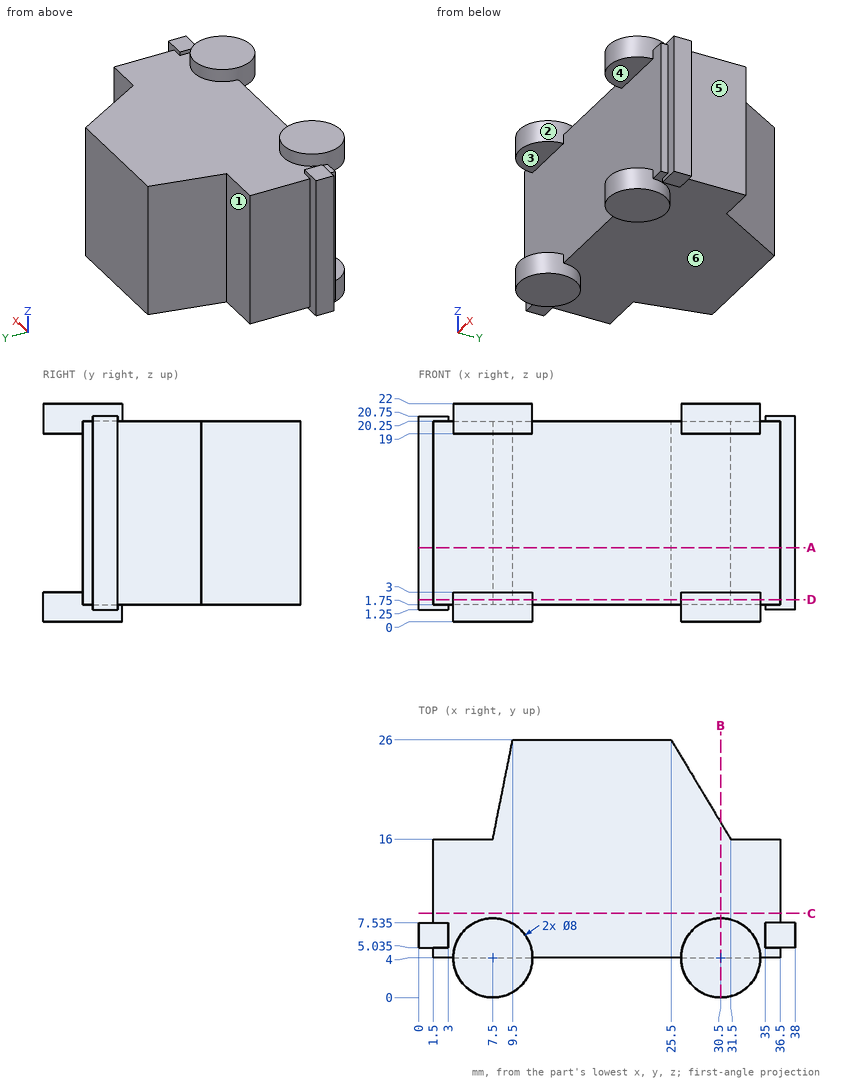
Input: dimensioned drawing with shaded views. Units: mm. Origin: part minimum x, y, z. A direction names the side the tool comes from. Coordinates: 2 decimals unless noted, no trailing zeros. Order: outer loops, then holes, each group sorted by start corner. A loop starts at its lowest first (then second) coordinate and runs counter-clockwise, first axis right, second up.
(1) Section query A-A (z = 7.5). Return the cut outline in (x, y) (1 decimal), plus the area to 4 significant figures.
(2) Draft query along X for the marked faces 4, 5 and 6. Return one class per face: pulls with the +X half, pulls with the -X half, needs draft (parallel to the pull), parting line crosses it, or undercut.
(3) Material intervals for probe 1 along Y at (x, z) = (17, 4); probe 2 along Z at (x, y) = (33.5, 8.5); probe 3 along Y at (x, z) = (35.5, 19.5), sorted ascending.
(4) Section query C-C (y = 8.5). Return the cut outline in (x, z), plus the area to 4 significant figures.
(5) Access query for the marked faces 1, 2 and 3. Directions: +Z, -Z, +X, -X, +Y, -Y. A direction counts if a zero-diameter tool reaches every point of the face in a straight line with its end or side. Return the directions, or none.
(6) Section query B-B (x = 30.5). Return the cut outline in (y, z).
(7) First-contact query: pin 1 (12 mm diameter, centred on x = 16.5, z = 11, fed in from -Y); pin 2 (3 mm diameter, centred on y = 19, z = 5, fed in from -X); pin 3 (2.5 mm diameter, centred on x = 36.5, z = 15.5, fed in from +Y). Flat tips, straight axial feed; report the tip coordinate or a pass-through.
(8) Section query D-D (z = 2.25). Return the cut outline in (x, y) (1 decimal).
Solution:
1. outline: (0, 5) - (1.5, 5) - (1.5, 4) - (36.5, 4) - (36.5, 5) - (38, 5) - (38, 7.5) - (36.5, 7.5) - (36.5, 16) - (31.5, 16) - (25.5, 26) - (9.5, 26) - (7.5, 16) - (1.5, 16) - (1.5, 7.5) - (0, 7.5) - close
1. area: 627.5 mm2
2. face 4: needs draft
2. face 5: pulls with the +X half
2. face 6: undercut
3. probe 1: y = 4 to 26
3. probe 2: z = 1.75 to 20.25
3. probe 3: y = 4 to 16
4. outline: (1.5, 1.75) - (36.5, 1.75) - (36.5, 20.25) - (1.5, 20.25) - close
4. area: 647.5 mm2
5. face 1: +Z, -Z, -X, +Y
5. face 2: +Z
5. face 3: +X, -X, -Y
6. outline: (0, 0) - (8, 0) - (8, 1.75) - (17.67, 1.75) - (17.67, 20.25) - (8, 20.25) - (8, 22) - (0, 22) - (0, 19) - (4, 19) - (4, 3) - (0, 3) - close
7. pin 1: stops at y = 4
7. pin 2: stops at x = 7.8
7. pin 3: stops at y = 16
8. outline: (0, 5) - (1.5, 5) - (1.5, 4) - (3.5, 4) arc R4 ccw to (11.5, 4) - (26.5, 4) arc R4 ccw to (34.5, 4) - (36.5, 4) - (36.5, 5) - (38, 5) - (38, 7.5) - (36.5, 7.5) - (36.5, 16) - (31.5, 16) - (25.5, 26) - (9.5, 26) - (7.5, 16) - (1.5, 16) - (1.5, 7.5) - (0, 7.5) - close
